```python
from build123d import *

# Parameters (mm, degrees)
SKETCH1_W           = 25
SKETCH1_H           = 4
BOSS_EXTRUDE1_DEPTH = 10
SKETCH2_R           = 0.75
CUT_EXTRUDE1_DEPTH  = 17.132265805
SKETCH4_W           = 4
SKETCH4_H           = 2
CUT_EXTRUDE2_DEPTH  = 1


with BuildPart() as part:
    # Sketch1 → Boss-Extrude1 (new body)
    with BuildSketch(Plane.XY):
        Rectangle(SKETCH1_W, SKETCH1_H)
    extrude(amount=BOSS_EXTRUDE1_DEPTH)

    # Sketch2 → Cut-Extrude1 (cut, through all)
    with BuildSketch(Plane(origin=(0, 0, 0), x_dir=(-1, 0, 0), z_dir=(0, 0, -1))):
        with Locations((-11.25, 1.75)):
            Circle(SKETCH2_R)
        with Locations((-8.75, 1.75)):
            Circle(SKETCH2_R)
        with Locations((-6.25, 1.75)):
            Circle(SKETCH2_R)
        with Locations((-3.75, 1.75)):
            Circle(SKETCH2_R)
        with Locations((-1.25, 1.75)):
            Circle(SKETCH2_R)
        with Locations((1.25, 1.75)):
            Circle(SKETCH2_R)
        with Locations((3.75, 1.75)):
            Circle(SKETCH2_R)
        with Locations((6.25, 1.75)):
            Circle(SKETCH2_R)
        with Locations((8.75, 1.75)):
            Circle(SKETCH2_R)
        with Locations((11.25, 1.75)):
            Circle(SKETCH2_R)
    extrude(amount=-CUT_EXTRUDE1_DEPTH, mode=Mode.SUBTRACT)

    # Sketch4 → Cut-Extrude2 (cut)
    with BuildSketch(Plane(origin=(12.5, 0, 0), x_dir=(0, 0, -1), z_dir=(1, 0, 0))):
        with Locations((-5, -1)):
            Rectangle(SKETCH4_W, SKETCH4_H)
    cut_extrude2 = extrude(amount=-CUT_EXTRUDE2_DEPTH, mode=Mode.SUBTRACT)

    # Mirror1: Cut-Extrude2 across plane
    add(cut_extrude2.mirror(Plane(origin=(0, 0, 0), x_dir=(0, 0, 1), z_dir=(1, 0, 0))), mode=Mode.SUBTRACT)


solid = part.part
```
Here's how the part is built. I have some questions about the finished solid (model axes, mm). A direction names the side the tool comes from. Give positions to 0.01 mm unless a question says otherwise; leave off trailing zeros. Order: outer loops, then holes, each group sorted by start corner. A loop starts at its lowest first (then second) coordinate and runs counter-clockwise, first axis right, second up. Notation, with made-up numbers: M 44.25,10.5 L 95.25,10.5 A18 cw 95.25,43.5 Z; hole C -33.5,88.25 d1. An arc over 180 degrees is marked long. Use a Markdown table: item, result. Add a question column.
1. On a 3-axis mill with a long thin cutter (end or side, diameter ignored), from which of +Z, -Z, +X, -X, +Y, -Y can I reach the whole of each face in a straight line? I mean faces 5 (the flat face through (12, 0, 5)), 6 (the flat face through (-12, 0, 5)), 7 (the flat face through (5, 2, 5)). Say none if no direction works.
2. If we mould it in two halves opening along X, with no side actions, what happens to faces 1 (the flat face through (11.5, -1, 5)), 2 (the flat face through (-11.5, -1, 5)), 3 (the cylindrical face through (6.3, 1, 4.9)), 4 (the flat face through (0, -2, 5))? For each: +X half, -X half, draft (parallel to the pull), parting line (faces both ways), or undercut.
3. Suppose I cut it at D-D (x = -6). List the corners of the cut face in (y, z) for me.
4. Suppose I cut it at C-C (y = 1.75). Give the number of separate pieces and of enclosed holes in the cut face, and give its area (3 significant figures).
5. Suppose I cut it at B-B (y = -1.75). List the corners of the cut face in (x, z) for me, and give its area (3 significant figures).
6. I need wall thicknesses on probe 1 along X at (y, z) = (-0.6, 5.25); probe 2 along Y at (x, z) = (-6.75, 9.5); probe 3 along Y at (x, z) = (6.5, 2.5). Which ranges of each line are inside material? Lowest first, please. Write a range as from..to.
7. Suppose I cut it at A-A (z = 1). List the corners of the cut face in (x, y) for me.
8. For pin 1 Ø0.8 at (x, z) = (-12, 4) entering from -Y; pin 2 Ø0.6 at (y, z) = (-1, 6) entering from -X, each with a flat end and sliding along its axis, tell me the tip position at first contact or that it passes through.
Results list:
| question | item | result |
|---|---|---|
| 1 | face 5 | +X, -Y |
| 1 | face 6 | -X, -Y |
| 1 | face 7 | +Z, -Z, +X, -X, +Y |
| 2 | face 1 | +X half |
| 2 | face 2 | -X half |
| 2 | face 3 | undercut |
| 2 | face 4 | draft |
| 3 | outline | M -2,0 L 1.04,0 L 1.04,10 L -2,10 Z |
| 4 | separate pieces | 11 |
| 4 | enclosed holes | 0 |
| 4 | area | 100 mm² |
| 5 | outline | M -12.5,0 L 12.5,0 L 12.5,3 L 11.5,3 L 11.5,7 L 12.5,7 L 12.5,10 L -12.5,10 L -12.5,7 L -11.5,7 L -11.5,3 L -12.5,3 Z |
| 5 | area | 242 mm² |
| 6 | probe 1 | x = -11.5..11.5 |
| 6 | probe 2 | y = -2..1.19 |
| 6 | probe 3 | y = -2..1.04 |
| 7 | outline | M -12.5,-2 L 12.5,-2 L 12.5,2 L 11.96,2 A0.75 cw long 10.54,2 L 9.46,2 A0.75 cw long 8.04,2 L 6.96,2 A0.75 cw long 5.54,2 L 4.46,2 A0.75 cw long 3.04,2 L 1.96,2 A0.75 cw long 0.54,2 L -0.54,2 A0.75 cw long -1.96,2 L -3.04,2 A0.75 cw long -4.46,2 L -5.54,2 A0.75 cw long -6.96,2 L -8.04,2 A0.75 cw long -9.46,2 L -10.54,2 A0.75 cw long -11.96,2 L -12.5,2 Z |
| 8 | pin 1 | stops at y = 0 |
| 8 | pin 2 | stops at x = -11.5 |
